from build123d import *

# Parameters (mm, degrees)
BOSS_EXTRUDE1_DEPTH      = 15
SKETCH4_R                = 2.55
CUT_EXTRUDE1_DEPTH       = 311.78207799
CUT_EXTRUDE3_DEPTH       = 258.997698633
CUT_EXTRUDE3_DEPTH_BACK  = 3.5
SKETCH5_R                = 4.5
SKETCH6_R                = 5
CUT_EXTRUDE4_DEPTH       = 258.997698633
CUT_EXTRUDE5_DEPTH       = 4
SKETCH8_R                = 1.6
CUT_EXTRUDE6_DEPTH       = 246.866452571
CUT_EXTRUDE7_DEPTH       = 2.5
SKETCH10_W               = 50
SKETCH10_H               = 23
SKETCH10_W_2             = 45.759160871
BOSS_EXTRUDE2_DEPTH      = 23
CUT_EXTRUDE8_START       = -24
SKETCH11_R               = 7.6
CUT_EXTRUDE8_DEPTH       = 325.431928593
SKETCH12_R               = 4.5
CUT_EXTRUDE9_DEPTH       = 301.431928593
SKETCH13_R               = 4.5
CUT_EXTRUDE10_DEPTH      = 259.586180025
CUT_EXTRUDE11_DEPTH      = 12.5
CUT_EXTRUDE11_DEPTH_BACK = 12.5
SKETCH14_R               = 7.6


with BuildPart() as part:
    # Sketch1 → Boss-Extrude1 (new body)
    with BuildSketch(Plane(origin=(0, 0, 0), x_dir=(1, 0, 0), z_dir=(0, 1, 0))):
        Polygon((25, 0), (-25, 0), (-25, -80), (-109.75, -183.961915416), (-109.75, -219.5), (-74.211915416, -219.5), (-20, -152.998825191), (20, -152.998825191), (74.211915416, -219.5), (109.75, -219.5), (109.75, -183.961915416), (25, -80), align=None)
    extrude(amount=BOSS_EXTRUDE1_DEPTH)

    # Sketch4 → Cut-Extrude1 (cut, through all)
    with BuildSketch(Plane.ZY.offset(109.75)):
        with Locations((30, 7.5)):
            Circle(SKETCH4_R)
        with Locations((70, 7.5)):
            Circle(SKETCH4_R)
        with Locations((110, 7.5)):
            Circle(SKETCH4_R)
        with Locations((142.998825191, 7.5)):
            Circle(SKETCH4_R)
    extrude(amount=-CUT_EXTRUDE1_DEPTH, mode=Mode.SUBTRACT)

    # Sketch5 → Cut-Extrude3 (cut, two sides: drawn at the far end of the back side and taken through both)
    with BuildSketch(Plane.ZY.offset(25).offset(-CUT_EXTRUDE3_DEPTH_BACK)):
        with Locations(Location((30, 7.5, 0), (0, 0, 180))):
            Circle(SKETCH5_R)
        with Locations(Location((70, 7.5, 0), (0, 0, 180))):
            Circle(SKETCH5_R)
        with Locations(Location((110, 7.5, 0), (0, 0, 180))):
            Circle(SKETCH5_R)
        with Locations(Location((142.998825191, 7.5, 0), (0, 0, 180))):
            Circle(SKETCH5_R)
    extrude(amount=CUT_EXTRUDE3_DEPTH + CUT_EXTRUDE3_DEPTH_BACK, mode=Mode.SUBTRACT)

    # Sketch6 → Cut-Extrude4 (cut, through all)
    with BuildSketch(Plane(origin=(25, 0, 0), x_dir=(0, 0, -1), z_dir=(1, 0, 0))):
        with Locations((-142.998825191, 7.5)):
            Circle(SKETCH6_R)
        with Locations((-110, 7.5)):
            Circle(SKETCH6_R)
    extrude(amount=CUT_EXTRUDE4_DEPTH, mode=Mode.SUBTRACT)

    # Sketch7 → Cut-Extrude5 (cut)
    with BuildSketch(Plane(origin=(25, 0, 0), x_dir=(0, 0, -1), z_dir=(1, 0, 0))):
        Polygon((-34.734272207, 7.5), (-32.367136104, 3.4), (-27.632863896, 3.4), (-25.265727793, 7.5), (-27.632863896, 11.6), (-32.367136104, 11.6), align=None)
        Polygon((-74.734272207, 7.5), (-72.367136104, 3.4), (-67.632863896, 3.4), (-65.265727793, 7.5), (-67.632863896, 11.6), (-72.367136104, 11.6), align=None)
        Polygon((-114.734272207, 7.5), (-112.367136104, 3.4), (-107.632863896, 3.4), (-105.265727793, 7.5), (-107.632863896, 11.6), (-112.367136104, 11.6), align=None)
        Polygon((-147.733097398, 7.5), (-145.365961294, 3.4), (-140.631689087, 3.4), (-138.264552983, 7.5), (-140.631689087, 11.6), (-145.365961294, 11.6), align=None)
    extrude(amount=-CUT_EXTRUDE5_DEPTH, mode=Mode.SUBTRACT)

    # Sketch8 → Cut-Extrude6 (cut, through all)
    with BuildSketch(Plane(origin=(0, 15, 0), x_dir=(1, 0, 0), z_dir=(0, 1, 0))):
        with Locations(Location((0, -5.25, 0), (0, 0, 270))):
            Circle(SKETCH8_R)
        with Locations(Location((-104.5, -214.25, 0), (0, 0, 270))):
            Circle(SKETCH8_R)
        with Locations(Location((104.5, -214.25, 0), (0, 0, 270))):
            Circle(SKETCH8_R)
    extrude(amount=-CUT_EXTRUDE6_DEPTH, mode=Mode.SUBTRACT)

    # Sketch9 → Cut-Extrude7 (cut)
    with BuildSketch(Plane(origin=(0, 15, 0), x_dir=(1, 0, 0), z_dir=(0, 1, 0))):
        Polygon((-101.209103466, -214.25), (-102.854551733, -211.4), (-106.145448267, -211.4), (-107.790896534, -214.25), (-106.145448267, -217.1), (-102.854551733, -217.1), align=None)
        Polygon((101.209103466, -214.25), (102.854551733, -217.1), (106.145448267, -217.1), (107.790896534, -214.25), (106.145448267, -211.4), (102.854551733, -211.4), align=None)
        Polygon((3.290896534, -5.25), (1.645448267, -2.4), (-1.645448267, -2.4), (-3.290896534, -5.25), (-1.645448267, -8.1), (1.645448267, -8.1), align=None)
    extrude(amount=-CUT_EXTRUDE7_DEPTH, mode=Mode.SUBTRACT)

    # Sketch10 → Boss-Extrude2 (add)
    with BuildSketch(Plane.XZ):
        with Locations((0, 43.25)):
            Rectangle(SKETCH10_W, SKETCH10_H)
        with Locations((71.208820555, 176.25)):
            Rectangle(SKETCH10_W_2, SKETCH10_H)
        with Locations((-71.208820555, 176.25)):
            Rectangle(SKETCH10_W_2, SKETCH10_H)
    extrude(amount=BOSS_EXTRUDE2_DEPTH)

    # Sketch11 → Cut-Extrude8 (cut)
    with BuildSketch(Plane.ZY.offset(94.08840099).offset(CUT_EXTRUDE8_START)):
        with Locations(Location((176.25, -11.5, 0), (0, 0, 180))):
            Circle(SKETCH11_R)
    cut_extrude8 = extrude(amount=CUT_EXTRUDE8_DEPTH, mode=Mode.SUBTRACT)

    # Sketch12 → Cut-Extrude9 (cut, through all)
    with BuildSketch(Plane.ZY.offset(94.08840099)):
        with Locations((176.25, -11.5)):
            Circle(SKETCH12_R)
    extrude(amount=-CUT_EXTRUDE9_DEPTH, mode=Mode.SUBTRACT)

    # Mirror1: Cut-Extrude8 across plane
    add(cut_extrude8.mirror(Plane(origin=(0, 0, 0), x_dir=(0, 0, 1), z_dir=(1, 0, 0))), mode=Mode.SUBTRACT)

    # Sketch13 → Cut-Extrude10 (cut, through all)
    with BuildSketch(Plane.ZY.offset(25)):
        with Locations((43.25, -11.5)):
            Circle(SKETCH13_R)
    extrude(amount=-CUT_EXTRUDE10_DEPTH, mode=Mode.SUBTRACT)

    # Sketch14 → Cut-Extrude11 (cut, two sides: drawn at the far end of the back side and taken through both)
    with BuildSketch(Plane(origin=(0, 0, 0), x_dir=(0, 0, -1), z_dir=(1, 0, 0)).offset(-CUT_EXTRUDE11_DEPTH_BACK)):
        with Locations((-43.25, -11.5)):
            Circle(SKETCH14_R)
    extrude(amount=CUT_EXTRUDE11_DEPTH + CUT_EXTRUDE11_DEPTH_BACK, mode=Mode.SUBTRACT)


solid = part.part
The listing builds one solid part. Answer for the finished solid, in the listing's coordinates (mm). A direction names the side the tool comes from. Round coordinates to 2 decimals unless told otherwise and drop trailing zeros. Loops run counter-clockwise (first coordinate to the right, second up) from the corner with the lowest first, then second, coordinate; pieces in that order, holes last. Notation, with made-up numbers: M 57,0 L 81,0 A15 ccw 81,5 Z; hole C 20.5,45 d6. An arc over 180 degrees is marked long. Return JSON: item names as keys, results as strings.
Q1. Find the intervals of material crossed by line 1 along Y through (x, z) = (-24, 30); line 2 along X through (y, z) = (6.75, 214.25); line 3 along Y through (x, z) = (15, 43), in increasing order. Write a range as from..to.
Results list:
{"line 1": "y = 0..3, 12..15", "line 2": "x = -109.75..-106.1, -102.9..-69.93, 69.93..102.9, 106.1..109.75", "line 3": "y = -23..-15.99, -7.01..15"}
Q2. Find section B-B, the plane z = 176. State how many separate pieces and enclosed holes the cut face has, plus the area to 3 significant figures.
Results list:
{"separate pieces": "4", "enclosed holes": "0", "area": "2,920 mm2"}
Q3. Each of these flat-tipped pins is pushed along its axis until it touches: pin 1 Ø8 at (y, z) = (7.5, 143) entering from -X; pin 2 Ø18.5 at (y, z) = (-11.5, 180) entering from +X; pin 3 Ø4.5 at (y, z) = (-11, 40.5) entering from -X; pin 4 Ø8 at (y, z) = (-3.5, 184.5) entering from -X. Where does it stop, or does it pass through?
Results list:
{"pin 1": "stops at x = -21.5", "pin 2": "stops at x = 94.09", "pin 3": "stops at x = -25", "pin 4": "stops at x = -109.75"}
Q4. Find section A-A, the plane z = 43.25. Determine the outline of the cut face in (x, y).
Results list:
{"outline": "M -25,-23 L 25,-23 L 25,-16 L 12.5,-16 L 12.5,-19.1 L -12.5,-19.1 L -12.5,-16 L -25,-16 Z; M -25,-7 L -12.5,-7 L -12.5,-3.9 L 12.5,-3.9 L 12.5,-7 L 25,-7 L 25,15 L -25,15 Z"}
Q5. Find section D-D, the plane z = 89. Determine the outline of the cut face in (x, y), plus the area to 3 significant figures.
Results list:
{"outline": "M -32.34,0 L 32.34,0 L 32.34,15 L -32.34,15 Z", "area": "970 mm2"}
Q6. The mould has two halves that part along Z. Classify faces 1 (the face through (-59.36, -13.22, 180.41)), 2 (the face through (-109.75, 7, 201)), 3 (the face through (0, 7, 0)): released by +Z, released by -Z, zero draft, split by the parting line, or undercut.
Results list:
{"face 1": "undercut", "face 2": "zero draft", "face 3": "released by -Z"}
Q7. Which of the six approach directions +Z, -Z, +X, -X, +Y, -Y give full straight-line access (tool end or side, diameter ignored) to faces 4 (the face through (21, 9.4, 108)), 5 (the face through (-103, 12.5, 213)), 6 (the face through (-21.5, 9.44, 28.06)), 7 (the face through (0, -11, 54.75))?
Results list:
{"face 4": "+X", "face 5": "+Y", "face 6": "-X", "face 7": "+Z, +X, -X, -Y"}
